Verification items for the finished model (mm, model axes). Coordinates: 2 decimals unless noted, no trailing zeros. Order: outer loops, then holes, each group sorted by start corner. A loop starts at its lowest first (then second) coordinate and runs counter-clockwise, first axis right, second up. Notation, with made-up numbers: M -34.75,75.25 L -27.75,75.25 A14 ccw -27.75,85.25 Z; hole C 19,-3.5 d7. An arc over 180 degrees is marked long. Answer as a JSON object with one key per item and string values. Group by question number.
(1) Gauge pin test, flat end, axial feed: pin 1 Ø1.5 at (x, y) = (111.5, -0.5) entering from +Z. Record the tip position at first contact, or that the pin passes through.
(2) Material ranges on line 1 (Z direction, x = -6, y = 1.4); line 2 (X direction, y = -0.8, z = -169); line 3 (Z direction, x = -105, y = 0.8), recorded low to high.
(3) Cross-section at C-C (y = 0.8). Count the separate pieces of the cut face and the enclosed holes in it, plus the area to 3 significant figures.
(4) Cross-section at A-A (x = -9). Enter the section's corners in (y, z), plus the area to 3 significant figures.
(5) Cross-section at B-B (z = -85). Enter the section's corners in (x, y).
from build123d import *

# Parameters (mm, degrees)
SKETCH1_W           = 236.5
SKETCH1_H           = 400
BOSS_EXTRUDE1_DEPTH = 1.5
FILLET1_R           = 30
SKETCH2_W           = 3
SKETCH2_H           = 30
CUT_EXTRUDE1_DEPTH  = 233.361921364
SKETCH3_W           = 30
SKETCH3_H           = 3
CUT_EXTRUDE2_DEPTH  = 233.361921364
CUT_EXTRUDE3_DEPTH  = 233.361921364


with BuildPart() as part:
    # Sketch1 → Boss-Extrude1 (new, symmetric)
    with BuildSketch(Plane(origin=(0, 0, 0), x_dir=(1, 0, 0), z_dir=(0, 1, 0))):
        Rectangle(SKETCH1_W, SKETCH1_H)
    extrude(amount=BOSS_EXTRUDE1_DEPTH, both=True)

    # Fillet1
    fillet1_edges = [part.edges().sort_by_distance(p)[0] for p in [
        (118.25, 0, 200),
        (-118.25, 0, 200),
        (-118.25, 0, -200),
        (118.25, 0, -200),
    ]]
    fillet(fillet1_edges, radius=FILLET1_R)

    # Sketch2 → Cut-Extrude1 (cut, through all)
    with BuildSketch(Plane(origin=(0, 1.5, 0), x_dir=(1, 0, 0), z_dir=(0, 1, 0))):
        with Locations((-111.75, -155)):
            Rectangle(SKETCH2_W, SKETCH2_H)
        with Locations((-111.75, -77.5)):
            Rectangle(SKETCH2_W, SKETCH2_H)
        with Locations((-111.75, 0)):
            Rectangle(SKETCH2_W, SKETCH2_H)
        with Locations((-111.75, 77.5)):
            Rectangle(SKETCH2_W, SKETCH2_H)
        with Locations((-111.75, 155)):
            Rectangle(SKETCH2_W, SKETCH2_H)
    cut_extrude1 = extrude(amount=-CUT_EXTRUDE1_DEPTH, mode=Mode.SUBTRACT)

    # Sketch3 → Cut-Extrude2 (cut, through all)
    with BuildSketch(Plane(origin=(0, 1.5, 0), x_dir=(1, 0, 0), z_dir=(0, 1, 0))):
        with Locations((-73.25, 193.5)):
            Rectangle(SKETCH3_W, SKETCH3_H)
        with Locations((0, 193.5)):
            Rectangle(SKETCH3_W, SKETCH3_H)
        with Locations((73.25, 193.5)):
            Rectangle(SKETCH3_W, SKETCH3_H)
    cut_extrude2 = extrude(amount=-CUT_EXTRUDE2_DEPTH, mode=Mode.SUBTRACT)

    # Mirror1: Cut-Extrude2 across plane
    add(cut_extrude2.mirror(Plane.XY), mode=Mode.SUBTRACT)

    # Mirror2: Cut-Extrude1 across plane
    add(cut_extrude1.mirror(Plane(origin=(0, 0, 0), x_dir=(0, 0, 1), z_dir=(1, 0, 0))), mode=Mode.SUBTRACT)

    # Sketch4 → Cut-Extrude3 (cut, through all)
    with BuildSketch(Plane(origin=(0, 1.5, 0), x_dir=(1, 0, 0), z_dir=(0, 1, 0))):
        Polygon((-108.756096654, 184.849242405), (-103.099242405, 190.506096654), (-100.718631416, 188.125485666), (-106.375485666, 182.468631416), align=None)
        Polygon((100.718631416, 188.125485666), (106.375485666, 182.468631416), (108.756096654, 184.849242405), (103.099242405, 190.506096654), align=None)
        Polygon((103.099242405, -190.506096654), (100.718631416, -188.125485666), (106.375485666, -182.468631416), (108.756096654, -184.849242405), align=None)
        Polygon((-100.718631416, -188.125485666), (-106.375485666, -182.468631416), (-108.756096654, -184.849242405), (-103.099242405, -190.506096654), align=None)
    extrude(amount=-CUT_EXTRUDE3_DEPTH, mode=Mode.SUBTRACT)


solid = part.part
Taken from the geometry:
{
 "1": {"pin 1": "stops at z = 189.84"},
 "2": {"line 1": "z = -200 to -195, -192 to 192, 195 to 200", "line 2": "x = -118.25 to -113.25, -110.25 to 110.25, 113.25 to 118.25", "line 3": "z = -194.89 to -188.61, -183.84 to 183.84, 188.61 to 194.89"},
 "3": {"separate pieces": "1", "enclosed holes": "20", "area": "92,300 mm²"},
 "4": {"outline": "M -1.5,-200 L 1.5,-200 L 1.5,-195 L -1.5,-195 Z; M -1.5,-192 L 1.5,-192 L 1.5,192 L -1.5,192 Z; M -1.5,195 L 1.5,195 L 1.5,200 L -1.5,200 Z", "area": "1,180 mm²"},
 "5": {"outline": "M -118.25,-1.5 L -113.25,-1.5 L -113.25,1.5 L -118.25,1.5 Z; M -110.25,-1.5 L 110.25,-1.5 L 110.25,1.5 L -110.25,1.5 Z; M 113.25,-1.5 L 118.25,-1.5 L 118.25,1.5 L 113.25,1.5 Z"}
}
